Model file for the job. Use its own axes, mm. A direction names the side the tool comes from. Round coordinates to 2 decimals unless told otherwise and drop trailing zeros. Loops run counter-clockwise (first coordinate to the right, second up) from the corner with the lowest first, then second, coordinate; pieces in that order, holes last. Notation, with made-up numbers: M 35,11 L 62,11 A25 ccw 62,36 Z; hole C -18,19.5 d4. An arc over 180 degrees is marked long. Use a Markdown table: item, result. Add a question column.
Q1. Cut at A-A (x = 8). Give the cut face in (y, z), plus the area to 3 significant figures.
Q2. Tool access for faces 1 (the face through (-3, 4, 1.25)), 2 (the face through (-4.2, 2, 0)), 3 (the face through (-3, 4, -1.25)): list every direction of +Z, -Z, +X, -X, +Y, -Y with a clear straight run to the whole face (end or side of a thin tool).
Q3. Pin check, flat tips, straight feed: pin 1 (1.3 mm diameter, centred on y = -1.5, z = 0.5, fed in from -X); pin 2 (4 mm diameter, centred on x = -5, y = -8, fed in from +Z); pin 3 (1.5 mm diameter, centred on x = -3, y = 3.5, fed in from +Z). Stop position of each tip, or through.
Q4. Cut at C-C (z = 0). State how many separate pieces and enclosed holes the cut face has, plus the area to 3 significant figures.
Q5. Cut at D-D (x = 4.25). Give the cut face in (y, z), plus the area to 3 significant figures.
Q6. Probe line 1 (X direction, y = 1.25, z = 0); line 2 (X direction, y = 0.75, z = -0.9); line 3 (Y direction, x = 4.75, z = 2.3). List the from-to ranges inside material, lowest first. Write a range as from..to.
Q7. Mould opens along X. For faces 4 (the face through (4.5, -1, 0)), 5 (the face through (9.86, 1, 0)), 6 (the face through (3, -8, 0.4)) say: +X half, -X half, draft (parallel to the pull), parting line (faces both ways), or undercut.
Q8. Cut at B-B (z = 2). Give the cut face in (x, y), plus the area to 3 significant figures.
from build123d import *

# Parameters (mm, degrees)
SKETCH1_W               = 19.72
SKETCH1_H               = 5.82
SKETCH1_R               = 1
BOSS_EXTRUDE1_DEPTH     = 2
SKETCH1_3_W             = 10.54
SKETCH1_3_H             = 5.82
BOSS_EXTRUDE2_DEPTH     = 4.4
CUT_EXTRUDE1_DEPTH      = 12.182472893
CUT_EXTRUDE1_DEPTH_BACK = 3
SKETCH1_4_W             = 9
SKETCH1_4_H             = 2.5
BOSS_EXTRUDE3_START     = -3
SKETCH1_5_W             = 3
SKETCH1_5_H             = 2.5
BOSS_EXTRUDE3_DEPTH     = 5
BOSS_EXTRUDE4_START     = 2
SKETCH1_6_W             = 3
SKETCH1_6_H             = 2.5
BOSS_EXTRUDE4_DEPTH     = 5
BOSS_EXTRUDE5_START     = -4.4
SKETCH2_W               = 2
SKETCH2_H               = 0.8
BOSS_EXTRUDE5_DEPTH     = 6.32
FILLET1_R               = 0.5


with BuildPart() as part:
    # Sketch1 → Boss-Extrude1 (new body)
    with BuildSketch(Plane(origin=(0, 0, 0), x_dir=(1, 0, 0), z_dir=(0, 1, 0))):
        Rectangle(SKETCH1_W, SKETCH1_H)
        with Locations(Location((8, 0, 0), (0, 0, 270))):
            Circle(SKETCH1_R, mode=Mode.SUBTRACT)
        with Locations(Location((-8, 0, 0), (0, 0, 270))):
            Circle(SKETCH1_R, mode=Mode.SUBTRACT)
    extrude(amount=BOSS_EXTRUDE1_DEPTH)

    # Sketch1<3> → Boss-Extrude2 (add)
    with BuildSketch(Plane(origin=(0, 0, 0), x_dir=(1, 0, 0), z_dir=(0, 1, 0))):
        Rectangle(SKETCH1_3_W, SKETCH1_3_H)
    extrude(amount=-BOSS_EXTRUDE2_DEPTH)

    # Sketch1<4> → Cut-Extrude1 (cut, two sides: drawn at the far end of the back side and taken through both)
    with BuildSketch(Plane(origin=(0, 0, 0), x_dir=(1, 0, 0), z_dir=(0, 1, 0)).offset(-CUT_EXTRUDE1_DEPTH_BACK)):
        Rectangle(SKETCH1_4_W, SKETCH1_4_H)
    extrude(amount=CUT_EXTRUDE1_DEPTH + CUT_EXTRUDE1_DEPTH_BACK, mode=Mode.SUBTRACT)

    # Sketch1<5> → Boss-Extrude3 (add)
    with BuildSketch(Plane(origin=(0, 0, 0), x_dir=(1, 0, 0), z_dir=(0, 1, 0)).offset(BOSS_EXTRUDE3_START)):
        with Locations((-2.7, 0)):
            Rectangle(SKETCH1_5_W, SKETCH1_5_H)
    extrude(amount=BOSS_EXTRUDE3_DEPTH)

    # Sketch1<6> → Boss-Extrude4 (add)
    with BuildSketch(Plane(origin=(0, 0, 0), x_dir=(1, 0, 0), z_dir=(0, 1, 0)).offset(BOSS_EXTRUDE4_START)):
        with Locations((-2.7, 0)):
            Rectangle(SKETCH1_6_W, SKETCH1_6_H)
    extrude(amount=BOSS_EXTRUDE4_DEPTH)

    # Sketch2 → Boss-Extrude5 (add)
    with BuildSketch(Plane(origin=(0, 0, 0), x_dir=(1, 0, 0), z_dir=(0, 1, 0)).offset(BOSS_EXTRUDE5_START)):
        with Locations((-2.8, 0)):
            Rectangle(SKETCH2_W, SKETCH2_H)
        Rectangle(SKETCH2_W, SKETCH2_H)
        with Locations((2.8, 0)):
            Rectangle(SKETCH2_W, SKETCH2_H)
    extrude(amount=-BOSS_EXTRUDE5_DEPTH)

    # Fillet1
    fillet1_edges = [part.edges().sort_by_distance(p)[0] for p in [
        (1.8, -10.72, 0),
        (3.8, -10.72, 0),
        (-3.8, -10.72, 0),
        (-1.8, -10.72, 0),
        (-1, -10.72, 0),
        (1, -10.72, 0),
    ]]
    fillet(fillet1_edges, radius=FILLET1_R)


solid = part.part
Checked values:
| question | item | result |
|---|---|---|
| 1 | outline | M 0,-2.91 L 2,-2.91 L 2,-1 L 0,-1 Z; M 0,1 L 2,1 L 2,2.91 L 0,2.91 Z |
| 1 | area | 7.64 mm^2 |
| 2 | face 1 | +Z, +X, -X, +Y |
| 2 | face 2 | +Y |
| 2 | face 3 | -Z, +X, -X, +Y |
| 3 | pin 1 | stops at x = -5.27 |
| 3 | pin 2 | stops at z = 0.4 |
| 3 | pin 3 | stops at z = 1.25 |
| 4 | separate pieces | 3 |
| 4 | enclosed holes | 0 |
| 4 | area | 100 mm^2 |
| 5 | outline | M -4.4,-2.91 L 2,-2.91 L 2,-1.25 L -3,-1.25 L -3,1.25 L 2,1.25 L 2,2.91 L -4.4,2.91 Z |
| 5 | area | 24.7 mm^2 |
| 6 | line 1 | x = -9.86..-9, -7..-4.5, -4.2..-1.2, 4.5..7, 9..9.86 |
| 6 | line 2 | x = -9.86..-8.44, -7.56..-4.5, -4.2..-1.2, 4.5..7.56, 8.44..9.86 |
| 6 | line 3 | y = -4.4..2 |
| 7 | face 4 | undercut |
| 7 | face 5 | +X half |
| 7 | face 6 | draft |
| 8 | outline | M -9.86,0 L -5.27,0 L -5.27,-4.4 L 5.27,-4.4 L 5.27,0 L 9.86,0 L 9.86,2 L -9.86,2 Z |
| 8 | area | 85.8 mm^2 |
